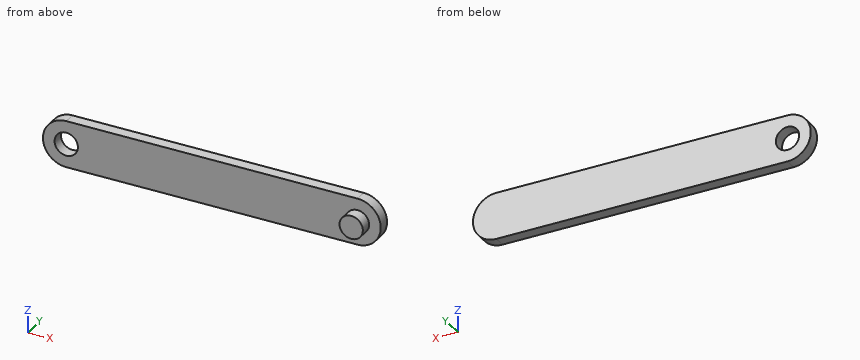
```python
from build123d import *

# Parameters (mm, degrees)
SKETCH1_R           = 1
BOSS_EXTRUDE2_DEPTH = 1
SKETCH5_R           = 1
BOSS_EXTRUDE3_DEPTH = 1


with BuildPart() as part:
    # Sketch1 → Boss-Extrude2 (new body)
    with BuildSketch(Plane(origin=(0, 0, 0), x_dir=(1, 0, 0), z_dir=(0, 1, 0))):
        with BuildLine():
            Line((-12.5, 2), (12.5, 2))
            ThreePointArc((12.5, 2), (14.5, 0), (12.5, -2))
            Line((12.5, -2), (-12.5, -2))
            ThreePointArc((-12.5, -2), (-14.5, 0), (-12.5, 2))
        make_face()
        with Locations((-12.5, 0)):
            Circle(SKETCH1_R, mode=Mode.SUBTRACT)
    extrude(amount=BOSS_EXTRUDE2_DEPTH)

    # Sketch5 → Boss-Extrude3 (add)
    with BuildSketch(Plane.XZ):
        with Locations((12.5, 0)):
            Circle(SKETCH5_R)
    extrude(amount=BOSS_EXTRUDE3_DEPTH)


solid = part.part
```
CAD build for the part. Positions are in the model's coordinates, mm. Coordinates: 2 decimals unless noted, no trailing zeros. Write each loop counter-clockwise with the first axis right and the second up, starting at its lowest first coordinate (ties: lowest second). Pieces come first, ordered by that corner, then holes. Notation, with made-up numbers: (79, 73.25) -> (126, 73.25) arc R18 ccw to (126, 104.25) -> close; hole circle Ø3 at (84, 77.25). An arc over 180 degrees is marked (long way). Return JSON: item names as keys, results as strings. Group by question number.
Q1. Cut at C-C, the plane x = 7. Give the cut face in (y, z), then the cut area to 3 significant figures.
Q2. Cut at D-D, the plane y = -0.6. Give the cut face in (x, z).
Q3. Flat gauge pins, fed straight in: pin 1 (1 mm diameter, centred on y = 0, z = 1.5, fed in from +X); pin 2 (1.2 mm diameter, centred on x = -12.5, z = 0, fed in from -Y). Where does each tip first touch, or does it go through?
Q4. Drill centre lines: line 1 (X direction, y = 0.85, z = 0); line 2 (Z direction, x = -12.5, y = 0.45); line 3 (Y direction, x = -1, z = -1.45). Where is each one in solid material? Low to high.
Q5. Cut at B-B, the plane z = 0.35. Give the cut face in (x, y).
Q6. Cut at A-A, the plane y = 0.45. Give the cut face in (x, z), then the cut area to 3 significant figures.
Returned:
{
 "1": {"outline": "(0, -2) -> (1, -2) -> (1, 2) -> (0, 2) -> close", "area": "4.00 mm2"},
 "2": {"outline": "circle Ø2 at (12.5, 0)"},
 "3": {"pin 1": "stops at x = 14.23", "pin 2": "passes through"},
 "4": {"line 1": "x = -14.5 to -13.5, -11.5 to 14.5", "line 2": "z = -2 to -1, 1 to 2", "line 3": "y = 0 to 1"},
 "5": {"outline": "(-14.47, 0) -> (-13.44, 0) -> (-13.44, 1) -> (-14.47, 1) -> close; (-11.56, 0) -> (11.56, 0) -> (11.56, -1) -> (13.44, -1) -> (13.44, 0) -> (14.47, 0) -> (14.47, 1) -> (-11.56, 1) -> close"},
 "6": {"outline": "(-12.5, -2) -> (12.5, -2) arc R2 ccw to (12.5, 2) -> (-12.5, 2) arc R2 ccw to start; hole circle Ø2 at (-12.5, 0)", "area": "109 mm2"}
}
